Verification items for the finished model (mm, model axes). Round coordinates to 2 decimals unless told otherwise and drop trailing zeros. Write each loop counter-clockwise with the first axis right and the second up, starting at its lowest first coordinate (ties: lowest second). Pieces come first, ordered by that corner, then holes. Notation, with made-up numbers: (-10.5, 68) -> (7.5, 68) arc R5 ccw to (7.5, 74) -> close; hole circle Ø8 at (58, -16.5). An arc over 180 degrees is marked (long way). Use CSV: the item, a comma, the result in double quotes.
```python
from build123d import *

# Parameters (mm, degrees)
SCHIZZO1_R                   = 219
SCHIZZO1_R_2                 = 176
SCHIZZO1_R_3                 = 7
ESTRUSIONE_ESTRUSIONE1_DEPTH = 2.5


with BuildPart() as part:
    # Schizzo1 → Estrusione-Estrusione1 (new, symmetric)
    with BuildSketch(Plane(origin=(0, 0, 0), x_dir=(1, 0, 0), z_dir=(0, 1, 0))):
        with Locations(Location((0, 0, 0), (0, 0, 270))):
            Circle(SCHIZZO1_R)
        with Locations(Location((0, 0, 0), (0, 0, 270))):
            Circle(SCHIZZO1_R_2, mode=Mode.SUBTRACT)
        with Locations(Location((0, 200, 0), (0, 0, 270))):
            Circle(SCHIZZO1_R_3, mode=Mode.SUBTRACT)
        with Locations(Location((141.421356237, 141.421356237, 0), (0, 0, 270))):
            Circle(SCHIZZO1_R_3, mode=Mode.SUBTRACT)
        with Locations(Location((200, 0, 0), (0, 0, 270))):
            Circle(SCHIZZO1_R_3, mode=Mode.SUBTRACT)
        with Locations(Location((141.421356237, -141.421356237, 0), (0, 0, 270))):
            Circle(SCHIZZO1_R_3, mode=Mode.SUBTRACT)
        with Locations(Location((0, -200, 0), (0, 0, 270))):
            Circle(SCHIZZO1_R_3, mode=Mode.SUBTRACT)
        with Locations(Location((-141.421356237, -141.421356237, 0), (0, 0, 270))):
            Circle(SCHIZZO1_R_3, mode=Mode.SUBTRACT)
        with Locations(Location((-200, 0, 0), (0, 0, 270))):
            Circle(SCHIZZO1_R_3, mode=Mode.SUBTRACT)
        with Locations(Location((-141.421356237, 141.421356237, 0), (0, 0, 270))):
            Circle(SCHIZZO1_R_3, mode=Mode.SUBTRACT)
    extrude(amount=ESTRUSIONE_ESTRUSIONE1_DEPTH, both=True)


solid = part.part
```
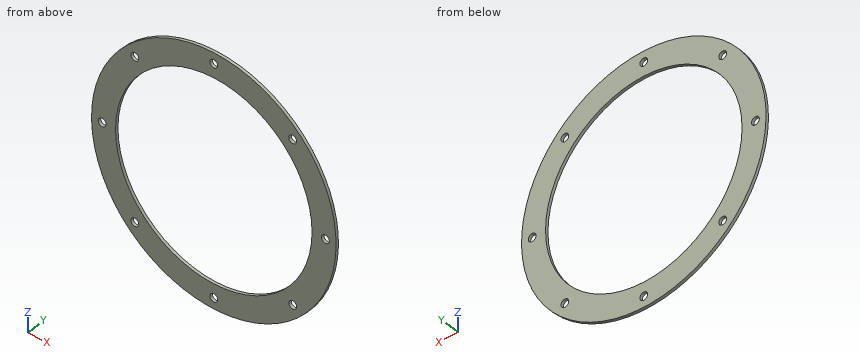
Q1. Go/stop test with flat-tipped pins: P1, Ø8.5, axis at x = 200, z = 0, coming from the +Y side; P2, Ø18, axis at x = 141.42, z = -141.42, coming from the +Y side; P3, Ø1, axis at y = 1.5, z = -104, coming from the +X side; P4, Ø1.5, axis at y = -2, z = 65.5, coming from the -X side. Record where each tip stops, or that it passes through.
Filled in:
P1,"through"
P2,"y = 2.5"
P3,"x = 193"
P4,"x = -209.21"
Q2. Section check A-A (z = 0). Record the cut outline in (x, y), plus the area to 3 significant figures.
Filled in:
outline,"(-219, -2.5) -> (-207, -2.5) -> (-207, 2.5) -> (-219, 2.5) -> close; (-193, -2.5) -> (-176, -2.5) -> (-176, 2.5) -> (-193, 2.5) -> close; (176, -2.5) -> (193, -2.5) -> (193, 2.5) -> (176, 2.5) -> close; (207, -2.5) -> (219, -2.5) -> (219, 2.5) -> (207, 2.5) -> close"
area,"290 mm²"
Q3. Section check C-C (z = -81). Record the cut outline in (x, y).
Filled in:
outline,"(-203.47, -2.5) -> (-156.25, -2.5) -> (-156.25, 2.5) -> (-203.47, 2.5) -> close; (156.25, -2.5) -> (203.47, -2.5) -> (203.47, 2.5) -> (156.25, 2.5) -> close"
Q4. Material ranges on L1, parallel to X at y = 0.1, z = 0; L2, parallel to Z at x = 152, y = -1; L3, parallel to X at y = 0.65, z = 200, recorded low to high.
Filled in:
L1,"-219 to -207, -193 to -176, 176 to 193, 207 to 219"
L2,"-157.66 to -88.72, 88.72 to 157.66"
L3,"-89.22 to -7, 7 to 89.22"
Q5. Section check D-D (y = 1). State how many separate pieces and enclosed holes the cut face has, plus the area to 3 significant figures.
Filled in:
separate pieces,"1"
enclosed holes,"9"
area,"52,100 mm²"
Q6. Section check B-B (x = 0). Record the cut outline in (y, z), plus the area to 3 significant figures.
Filled in:
outline,"(-2.5, -219) -> (2.5, -219) -> (2.5, -207) -> (-2.5, -207) -> close; (-2.5, -193) -> (2.5, -193) -> (2.5, -176) -> (-2.5, -176) -> close; (-2.5, 176) -> (2.5, 176) -> (2.5, 193) -> (-2.5, 193) -> close; (-2.5, 207) -> (2.5, 207) -> (2.5, 219) -> (-2.5, 219) -> close"
area,"290 mm²"
